Build history of the part. All positions in model axes, mm. Coordinates: 2 decimals unless noted, no trailing zeros. Loops run counter-clockwise (first coordinate to the right, second up) from the corner with the lowest first, then second, coordinate; pieces in that order, holes last. Notation, with made-up numbers: (23, 0) - (82, 0) arc R8 cw to (82, 5) - close; hole circle Ø8 at (74, 11.25). An arc over 180 degrees is marked (long way). One line per item, written item: value.
```python
from build123d import *

# Parameters (mm, degrees)
EXTRUDE_1_DEPTH = 3


with BuildPart() as part:
    # Эскиз1 → Бобышка-Вытянуть1 (new body)
    with BuildSketch(Plane(origin=(0, 0, 0), x_dir=(1, 0, 0), z_dir=(0, 1, 0))):
        with BuildLine():
            Line((0, 15), (0, 10))
            ThreePointArc((0, 10), (2.5, 7.5), (0, 5))
            Line((0, 5), (0, 0))
            Line((0, 0), (10, 0))
            Line((10, 0), (10, 15))
            Line((10, 15), (0, 15))
        make_face()
    extrude(amount=EXTRUDE_1_DEPTH)


solid = part.part
```
Item 1: Cut at D-D, the plane z = -7.5. Write the cut outline in (x, y), then the cut area to 3 significant figures.
Check result:
outline: (2.5, 0) - (10, 0) - (10, 3) - (2.5, 3) - close
area: 22.5 mm^2
Item 2: Cut at C-C, the plane z = -9.5. Write the cut outline in (x, y).
Check result:
outline: (1.5, 0) - (10, 0) - (10, 3) - (1.5, 3) - close
Item 3: Cut at A-A, the plane x = 1.5. Write the cut outline in (y, z).
Check result:
outline: (0, -15) - (3, -15) - (3, -9.5) - (0, -9.5) - close; (0, -5.5) - (3, -5.5) - (3, 0) - (0, 0) - close
Item 4: Probe probe 1 along Z at (x, y) = (1.5, 1.35); probe 2 along X at (y, z) = (1.05, -5.25); probe 3 along Z at (x, y) = (0.75, 2.75). List the from-to ranges inside material, lowest first. Write a range as from..to.
Check result:
probe 1: z = -15..-9.5, -5.5..0
probe 2: x = 1.09..10
probe 3: z = -15..-9.88, -5.12..0
Item 5: Pull direction Z, two halves, no side cores. Call faces 1 (the face through (0, 1, -13)), 2 (the face through (5, 1, -15)), 3 (the face through (2.5, 1.5, -7.6)), 4 (the face through (5, 1, 0)): released by +Z, released by -Z, zero draft, split by the parting line, or undercut.
Check result:
face 1: zero draft
face 2: released by -Z
face 3: undercut
face 4: released by +Z
Item 6: Cut at B-B, the plane y = 2. Write the cut outline in (x, z).
Check result:
outline: (0, -15) - (10, -15) - (10, 0) - (0, 0) - (0, -5) arc R2.5 cw to (0, -10) - close
